Design review of the part built by this model. Coordinates are the model's own, in mm. Face numbers are marked on the shaded views. Coordinates: 2 decimals unless noted, no trailing zeros. Loops run counter-clockwise (first coordinate to the right, second up) from the corner with the lowest first, then second, coordinate; pieces in that order, holes last.
Q1. Add section B-B on y = 4.5. Give the number of separate pieces and of enclosed holes in the cut face, and give its area (3 significant figures).
Q2. For P1, Ø3, axis at y = 3.5, z = -123.5, coming from the +X side; P2, Ø3, axis at x = -74.5, y = 4, coming from the -Z side; P3, Ø3, axis at x = -1, y = 3.5, coming from the +Z side, all flat-tipped, find the tip position at first contact; note any pin that passes through.
Q3. Add section A-A on z = -64. Give the boundary of the cut face in (x, y), and give its area (3 significant figures).
Q4. Wall thickness on probe 1 along X at (y, z) = (3, 103); probe 2 along Z at (x, y) = (-23.5, 0.75); probe 3 along X at (y, z) = (0.75, 78): over which ranges is each line inside the solid? List them lowest first.
Q5. Draft analysis for pull direction Y (two halves, no side actions). For the marked faces 1 and 2, state which applies: released by +Y, released by -Y, zero draft, split by the parting line, or undercut.
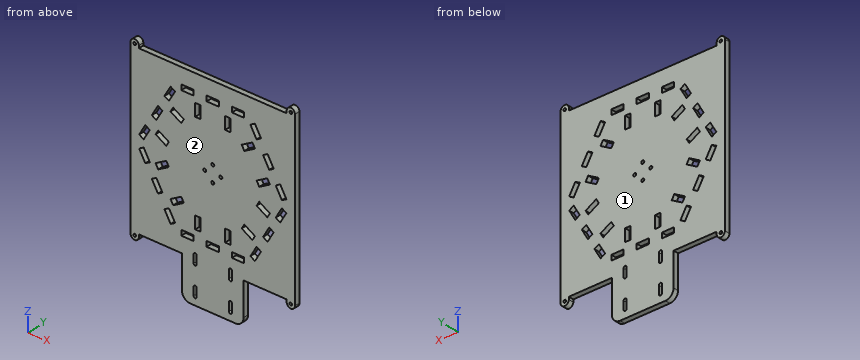
```python
from build123d import *

# Parameters (mm, degrees)
ESQUISSE1_W                     = 200
ESQUISSE1_H                     = 200
BOSS_EXTRU_1_DEPTH              = 6.35
BOSS_EXTRU_2_DEPTH              = 6.35
ENL_V_MAT_EXTRU_1_REACH         = 149.324
ESQUISSE3_R                     = 1.5875
R_P_TITION_LIN_AIRE1_COUNT      = 2
R_P_TITION_LIN_AIRE1_PITCH      = 190
SYM_TRIE1_COPY_1_DEPTH          = 6.35
SYM_TRIE1_COPY_2_REACH          = 149.324
SYM_TRIE1_COPY_2_SKETCH_R       = 1.5875
ESQUISSE4_W                     = 75
ESQUISSE4_H                     = 50
BOSS_EXTRU_3_DEPTH              = 6.35
CONG_1_R                        = 10
SKETCH1_R                       = 1.8288
CUT_EXTRUDE1_DEPTH              = 6.35
CIRPATTERN1_COUNT               = 4
ESQUISSE7_W                     = 15
ESQUISSE7_H                     = 6.35
ENL_V_MAT_EXTRU_2_DEPTH         = 6.35
R_P_TITION_CIRCULAIRE1_COUNT    = 6
ENL_V_MAT_EXTRU_3_REACH         = 182.389
R_P_TITION_LIN_AIRE2_COUNT      = 2
R_P_TITION_LIN_AIRE2_PITCH      = 35
R_P_TITION_LIN_AIRE2_COUNT_DIR2 = 2
R_P_TITION_LIN_AIRE2_PITCH_DIR2 = 43
ENL_V_MAT_EXTRU_4_REACH         = 182.389
ESQUISSE9_W                     = 6.35
ESQUISSE9_H                     = 15
R_P_TITION_CIRCULAIRE2_COUNT    = 6


with BuildPart() as part:
    # Esquisse1 → Boss.-Extru.1 (new body)
    with BuildSketch(Plane(origin=(0, 0, 0), x_dir=(1, 0, 0), z_dir=(0, 1, 0))):
        Rectangle(ESQUISSE1_W, ESQUISSE1_H)
    extrude(amount=BOSS_EXTRU_1_DEPTH)

    # Esquisse2 → Boss.-Extru.2 (add)
    with BuildSketch(Plane(origin=(0, 6.35, 0), x_dir=(1, 0, 0), z_dir=(0, 1, 0))):
        with BuildLine():
            Line((-100, 100), (-90, 100))
            Line((-90, 100), (-90, 103))
            ThreePointArc((-90, 103), (-95, 108), (-100, 103))
            Line((-100, 103), (-100, 100))
        make_face()
    boss_extru_2 = extrude(amount=-BOSS_EXTRU_2_DEPTH)

    # Esquisse3 → Enl_v. mat.-Extru.1 (cut, up to next)
    with BuildSketch(Plane(origin=(0, 6.35, 0), x_dir=(1, 0, 0), z_dir=(0, 1, 0)), mode=Mode.PRIVATE) as enl_v_mat_extru_1_sk1:
        with Locations(Location((-95, 103, 0), (0, 0, 270))):
            Circle(ESQUISSE3_R)
    enl_v_mat_extru_1_tool1 = extrude(enl_v_mat_extru_1_sk1.sketch, amount=-ENL_V_MAT_EXTRU_1_REACH, mode=Mode.PRIVATE) & part.part
    enl_v_mat_extru_1 = enl_v_mat_extru_1_tool1.solids().sort_by_distance((-95, 6.35, -103))[0]
    add(enl_v_mat_extru_1, mode=Mode.SUBTRACT)

    # R_p_tition lin_aire1: Boss.-Extru.2, Enl_v. mat.-Extru.1 ×2
    with Locations(*[(i * R_P_TITION_LIN_AIRE1_PITCH, 0, 0) for i in range(1, R_P_TITION_LIN_AIRE1_COUNT)]):
        add(boss_extru_2)
        add(enl_v_mat_extru_1, mode=Mode.SUBTRACT)

    # Sym_trie1: Boss.-Extru.2, Enl_v. mat.-Extru.1 across plane
    add(boss_extru_2.mirror(Plane.XY))
    add(enl_v_mat_extru_1.mirror(Plane.XY), mode=Mode.SUBTRACT)

    # Sym_trie1 copy 1 sketch → Sym_trie1 copy 1 (add)
    with BuildSketch(Plane(origin=(190, 6.35, 0), x_dir=(1, 0, 0), z_dir=(0, 1, 0))):
        with BuildLine():
            Line((-100, -100), (-90, -100))
            Line((-90, -100), (-90, -103))
            ThreePointArc((-90, -103), (-95, -108), (-100, -103))
            Line((-100, -103), (-100, -100))
        make_face()
    extrude(amount=-SYM_TRIE1_COPY_1_DEPTH)

    # Sym_trie1 copy 2 sketch → Sym_trie1 copy 2 (cut, up to next)
    with BuildSketch(Plane(origin=(190, 6.35, 0), x_dir=(1, 0, 0), z_dir=(0, 1, 0)), mode=Mode.PRIVATE) as sym_trie1_copy_2_sk1:
        with Locations((-95, -103)):
            Circle(SYM_TRIE1_COPY_2_SKETCH_R)
    sym_trie1_copy_2_tool1 = extrude(sym_trie1_copy_2_sk1.sketch, amount=-SYM_TRIE1_COPY_2_REACH, mode=Mode.PRIVATE) & part.part
    add(sym_trie1_copy_2_tool1.solids().sort_by_distance((95, 6.35, 103))[0], mode=Mode.SUBTRACT)

    # Esquisse4 → Boss.-Extru.3 (add)
    with BuildSketch(Plane(origin=(0, 6.35, 0), x_dir=(1, 0, 0), z_dir=(0, 1, 0))):
        with Locations((0, 125)):
            Rectangle(ESQUISSE4_W, ESQUISSE4_H)
    extrude(amount=-BOSS_EXTRU_3_DEPTH)

    # Cong_1
    cong_1_edges = [part.edges().sort_by_distance(p)[0] for p in [
        (-37.5, 3.175, -150),
        (37.5, 3.175, -150),
    ]]
    fillet(cong_1_edges, radius=CONG_1_R)

    # Sketch1 → Cut-Extrude1 (cut)
    with BuildSketch(Plane.XZ):
        with Locations(Location((0, -9.779, 0), (0, 0, 270))):
            Circle(SKETCH1_R)
    cut_extrude1 = extrude(amount=-CUT_EXTRUDE1_DEPTH, mode=Mode.SUBTRACT)

    # CirPattern1: Cut-Extrude1 ×4 about axis
    cirpattern1_axis = Axis((0, 0, 0), (0, 1, 0))
    for i in range(1, CIRPATTERN1_COUNT):
        add(cut_extrude1.rotate(cirpattern1_axis, i * 360 / CIRPATTERN1_COUNT), mode=Mode.SUBTRACT)

    # Esquisse7 → Enl_v. mat.-Extru.2 (cut)
    with BuildSketch(Plane.XZ):
        with Locations((30.801270189, -78.175)):
            Rectangle(ESQUISSE7_W, ESQUISSE7_H)
        with Locations((0, -78.175)):
            Rectangle(ESQUISSE7_W, ESQUISSE7_H)
        with Locations((-30.801270189, -78.175)):
            Rectangle(ESQUISSE7_W, ESQUISSE7_H)
    enl_v_mat_extru_2 = extrude(amount=-ENL_V_MAT_EXTRU_2_DEPTH, mode=Mode.SUBTRACT)

    # R_p_tition circulaire1: Enl_v. mat.-Extru.2 ×6 about axis
    r_p_tition_circulaire1_axis = Axis((0, 0, 0), (0, 1, 0))
    for i in range(1, R_P_TITION_CIRCULAIRE1_COUNT):
        add(enl_v_mat_extru_2.rotate(r_p_tition_circulaire1_axis, i * 360 / R_P_TITION_CIRCULAIRE1_COUNT), mode=Mode.SUBTRACT)

    # Esquisse8 → Enl_v. mat.-Extru.3 (cut, up to next)
    with BuildSketch(Plane(origin=(0, 6.35, 0), x_dir=(1, 0, 0), z_dir=(0, 1, 0)), mode=Mode.PRIVATE) as enl_v_mat_extru_3_sk1:
        with BuildLine():
            Line((-19.666666667, 140.227252842), (-19.666666667, 130.227252842))
            ThreePointArc((-19.666666667, 130.227252842), (-21.5, 128.393919509), (-23.333333333, 130.227252842))
            Line((-23.333333333, 130.227252842), (-23.333333333, 140.227252842))
            ThreePointArc((-23.333333333, 140.227252842), (-21.5, 142.060586175), (-19.666666667, 140.227252842))
        make_face()
    enl_v_mat_extru_3_tool1 = extrude(enl_v_mat_extru_3_sk1.sketch, amount=-ENL_V_MAT_EXTRU_3_REACH, mode=Mode.PRIVATE) & part.part
    enl_v_mat_extru_3 = enl_v_mat_extru_3_tool1.solids().sort_by_distance((-21.5, 6.35, -135.227253))[0]
    add(enl_v_mat_extru_3, mode=Mode.SUBTRACT)

    # R_p_tition lin_aire2: Enl_v. mat.-Extru.3 2 × 2
    with Locations(*[(j * R_P_TITION_LIN_AIRE2_PITCH_DIR2, 0, i * R_P_TITION_LIN_AIRE2_PITCH) for i in range(R_P_TITION_LIN_AIRE2_COUNT) for j in range(R_P_TITION_LIN_AIRE2_COUNT_DIR2) if (i, j) != (0, 0)]):
        add(enl_v_mat_extru_3, mode=Mode.SUBTRACT)

    # Esquisse9 → Enl_v. mat.-Extru.4 (cut, up to next)
    with BuildSketch(Plane.XZ, mode=Mode.PRIVATE) as enl_v_mat_extru_4_sk1:
        with Locations((-18.175, -60.5)):
            Rectangle(ESQUISSE9_W, ESQUISSE9_H)
    enl_v_mat_extru_4_tool1 = extrude(enl_v_mat_extru_4_sk1.sketch, amount=-ENL_V_MAT_EXTRU_4_REACH, mode=Mode.PRIVATE) & part.part
    # Esquisse9 → Enl_v. mat.-Extru.4 (cut, up to next)
    with BuildSketch(Plane.XZ, mode=Mode.PRIVATE) as enl_v_mat_extru_4_sk2:
        with Locations((18.175, -60.5)):
            Rectangle(ESQUISSE9_W, ESQUISSE9_H)
    enl_v_mat_extru_4_tool2 = extrude(enl_v_mat_extru_4_sk2.sketch, amount=-ENL_V_MAT_EXTRU_4_REACH, mode=Mode.PRIVATE) & part.part
    enl_v_mat_extru_4_1 = enl_v_mat_extru_4_tool1.solids().sort_by_distance((-18.175, 0, -60.5))[0]
    add(enl_v_mat_extru_4_1, mode=Mode.SUBTRACT)
    enl_v_mat_extru_4_2 = enl_v_mat_extru_4_tool2.solids().sort_by_distance((18.175, 0, -60.5))[0]
    add(enl_v_mat_extru_4_2, mode=Mode.SUBTRACT)
    enl_v_mat_extru_4 = enl_v_mat_extru_4_1 + enl_v_mat_extru_4_2  # Enl_v. mat.-Extru.4 as one shape, for the pattern or mirror that repeats it

    # R_p_tition circulaire2: Enl_v. mat.-Extru.4 ×6 about axis
    r_p_tition_circulaire2_axis = Axis((0, 0, 0), (0, 1, 0))
    for i in range(1, R_P_TITION_CIRCULAIRE2_COUNT):
        add(enl_v_mat_extru_4.rotate(r_p_tition_circulaire2_axis, i * 360 / R_P_TITION_CIRCULAIRE2_COUNT), mode=Mode.SUBTRACT)


solid = part.part
```
Entries:
1. separate pieces: 1
1. enclosed holes: 42
1. area: 40,900 mm2
2. P1: stops at x = 37.5
2. P2: stops at z = -100
2. P3: stops at z = 100
3. outline: (-100, 0) - (-56.98, 0) - (-56.98, 6.35) - (-100, 6.35) - close; (-49.65, 0) - (-21.35, 0) - (-21.35, 6.35) - (-49.65, 6.35) - close; (-15, 0) - (15, 0) - (15, 6.35) - (-15, 6.35) - close; (21.35, 0) - (49.65, 0) - (49.65, 6.35) - (21.35, 6.35) - close; (56.98, 0) - (100, 0) - (100, 6.35) - (56.98, 6.35) - close
3. area: 1,100 mm2
4. probe 1: x = -100 to -96.59, -93.41 to -90, 90 to 93.41, 96.59 to 100
4. probe 2: z = -150 to -81.35, -75 to 75, 81.35 to 100
4. probe 3: x = -100 to -38.3, -23.3 to -7.5, 7.5 to 23.3, 38.3 to 100
5. face 1: released by +Y
5. face 2: released by -Y
